Here's how the part is built. I have some questions about the finished solid (model axes, mm). Face numbers are marked on the shaded views. A direction names the side the tool comes from. Give positions to 0.01 mm unless a question says otherwise; leave off trailing zeros. Order: outer loops, then holes, each group sorted by start corner. A loop starts at its lowest first (then second) coordinate and runs counter-clockwise, first axis right, second up.
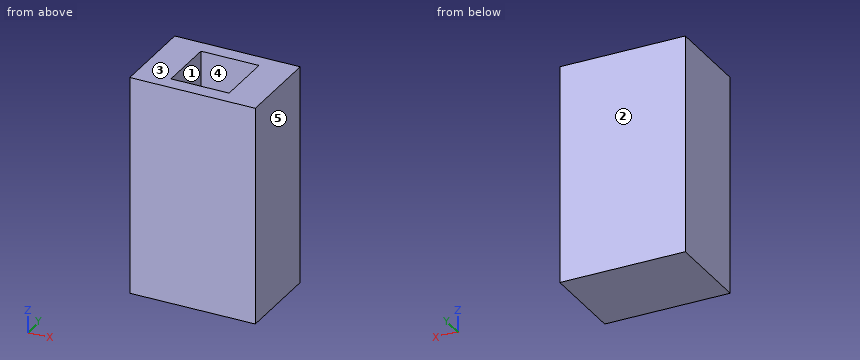
from build123d import *

# Parameters (mm, degrees)
SKETCH1_W           = 86.35
SKETCH1_H           = 60
BOSS_EXTRUDE1_DEPTH = 150
SKETCH2_W           = 40
SKETCH2_H           = 40
CUT_EXTRUDE1_DEPTH  = 145


with BuildPart() as part:
    # Sketch1 → Boss-Extrude1 (new body)
    with BuildSketch(Plane.XY):
        Rectangle(SKETCH1_W, SKETCH1_H)
    extrude(amount=BOSS_EXTRUDE1_DEPTH)

    # Sketch2 → Cut-Extrude1 (cut)
    with BuildSketch(Plane(origin=(0, 0, 150), x_dir=(-1, 0, 0), z_dir=(0, 0, -1))):
        Rectangle(SKETCH2_W, SKETCH2_H)
    extrude(amount=CUT_EXTRUDE1_DEPTH, mode=Mode.SUBTRACT)


solid = part.part
Q1. If we section it at A-A on z = 34: List the corners of the cut face in (x, y) for me (3 decimals).
Filled sheet:
outline: (-43.175, -30) - (43.175, -30) - (43.175, 30) - (-43.175, 30) - close; hole (-20, -20) - (20, -20) - (20, 20) - (-20, 20) - close
Q2. Thinking about a two-plate mould opening in X: for the marked faces 3, 4 and 5, which applies, released by +X, released by -X, zero draft, split by the parting line, or undercut?
Filled sheet:
face 3: zero draft
face 4: undercut
face 5: released by +X
Q3. If we section it at B-B on x = -7: List the corners of the cut face in (y, z) for me.
Filled sheet:
outline: (-30, 0) - (30, 0) - (30, 150) - (20, 150) - (20, 5) - (-20, 5) - (-20, 150) - (-30, 150) - close
Q4. For the marked faces 1 and 2, which set-ups out of +Z, -Z, +X, -X, +Y, -Y let a thin tool reach every point of the face, with its end or its side?
Filled sheet:
face 1: +Z
face 2: +Z, -Z, +X, -X, +Y
Q5. I need wall thicknesses on L1, parallel to X at y = -11.5, z = 79 (3 decimals); L2, parallel to Y at x = 15.5, z = 124; L3, parallel to Z at x = 12, y = -9. Which ranges of each line are inside material? Lowest first, please.
Filled sheet:
L1: x = -43.175 to -20, 20 to 43.175
L2: y = -30 to -20, 20 to 30
L3: z = 0 to 5
Q6. I'm going to push a flat-ended pin straight in: P1, Ø10, axis at x = 8.5, y = -1.5, coming from the +Z side. Where does the tip first touch, or does it pass through?
Filled sheet:
P1: stops at z = 5
Q7. If we section it at C-C on y = 0: List the corners of the cut face in (x, z) for me (3 decimals).
Filled sheet:
outline: (-43.175, 0) - (43.175, 0) - (43.175, 150) - (20, 150) - (20, 5) - (-20, 5) - (-20, 150) - (-43.175, 150) - close
